Geometry: final body of the model. Coordinates: model frame, mm. Face numbers are marked on the shaded views. A direction names the side the tool comes from. Give positions to 0.01 mm unless a question says otherwise; leave off trailing zeros. Write each loop counter-clockwise with the first axis right and the second up, starting at its lowest first coordinate (ties: lowest second). Pieces come first, ordered by that corner, then holes.
Q1. Section C-C (z = -1.5). Return the cut outline in (x, y).
Q2. Pin query (flat end, axial travel): pin 1 Ø12 at (x, y) = (74, -29.5) entering from +Z; pin 2 Ø6 at (y, z) = (-23, -5) entering from +X; pin 3 Ø0.9 at (x, y) = (95.5, -13.5) entering from -Z. Return the tip coordinate at first contact, or that it passes through.
Q3. Section D-D (y = -25). Return the cut outline in (x, z) (3 decimals), plus the area to 3 significant figures.
Q4. Section B-B (x = 55.5). Return the cut outline in (y, z).
Q5. Reachability of the marked faces 1 and 2 from +Z, -Z, +X, -X, +Y, -Y: full face, straight path, thin tool, end or side. Return the list, or none.
Q6. Line query: line 1 (Z direction, x = 44.5, y = -6.5); line 2 (Y direction, x = 22, z = -9.5); line 3 (Z direction, x = 97, y = -20). Output: solid intervals per line, ascending.
Q7. Section A-A (y = -53.5). Return the cut outline in (x, z), plus the area to 3 significant figures.
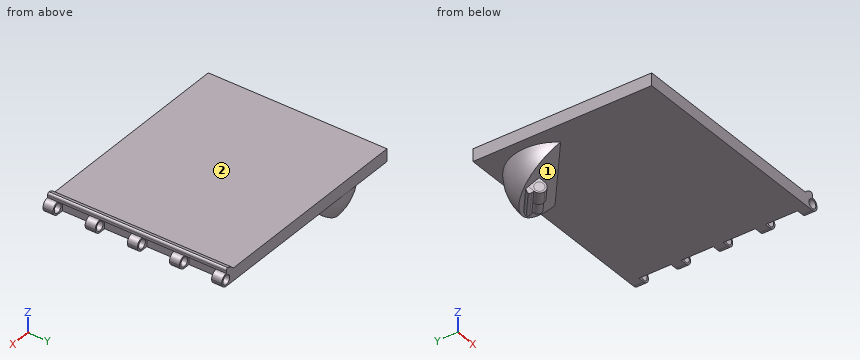
from build123d import *

# Parameters (mm, degrees)
F0_W      = 100
F0_H      = 5.6
F1_DEPTH  = 80
F3_R      = 2.05
F4_DEPTH  = 80
F2_W      = 5.7
F2_H      = 14.37
F2_W_2    = 5.6900524584
F2_W_3    = 5.6801049167
F2_W_4    = 5.6701573751
F5_DEPTH  = 5.6
F6_DEPTH  = 80
F8_ANGLE  = 45
F10_DEPTH = 5.6
F12_DEPTH = 7.185
F11_R     = 2.05
F13_DEPTH = 14.37


with BuildPart() as f1:
    # F0 (on Front) → F1 (new body)
    with BuildSketch(Plane.XZ):
        with Locations((50, 2.8)):
            Rectangle(F0_W, F0_H)
    extrude(amount=F1_DEPTH)

    # F3 (on face) → F4 (cut)
    with BuildSketch(Plane(origin=(0, 0, 0), x_dir=(-1, 0, 0), z_dir=(0, 1, 0))):
        with BuildLine():
            ThreePointArc((-100, 2.8), (-99.1798989873, 4.7798989873), (-97.2, 5.6))
            Line((-97.2, 5.6), (-100, 5.6))
            Line((-100, 5.6), (-100, 2.8))
        make_face()
        with BuildLine():
            ThreePointArc((-97.2, 0), (-99.1798989873, 0.8201010127), (-100, 2.8))
            Line((-100, 2.8), (-100, 0))
            Line((-100, 0), (-97.2, 0))
        make_face()
        with Locations((-97.2, 2.8)):
            Circle(F3_R)
    extrude(amount=-F4_DEPTH, mode=Mode.SUBTRACT)

    # F2 (on face) → F5 (cut)
    with BuildSketch(Plane.XY.offset(5.6)):
        with Locations((97.15, -11.689)):
            Rectangle(F2_W, F2_H)
        with Locations((97.1549737708, -30.5629973786)):
            Rectangle(F2_W_2, F2_H)
        with Locations((97.1599475416, -49.4369947571)):
            Rectangle(F2_W_3, F2_H)
        with Locations((97.1649213125, -68.3109921357)):
            Rectangle(F2_W_4, F2_H)
    extrude(amount=-F5_DEPTH, mode=Mode.SUBTRACT)

    # F3 (on face) → F6 (join)
    with BuildSketch(Plane(origin=(0, 0, 0), x_dir=(-1, 0, 0), z_dir=(0, 1, 0))):
        with BuildLine():
            ThreePointArc((-96.4487730361, 7.7432436768), (-96.9926506427, 7.3427867688), (-97.2, 6.7))
            ThreePointArc((-97.2, 6.7), (-96.8778174593, 5.9221825407), (-96.1, 5.6))
            Line((-96.1, 5.6), (-94.4, 5.6))
            Line((-94.4, 5.6), (-93.0575369646, 5.6))
            ThreePointArc((-93.0575369646, 5.6), (-94.5287785908, 7.0266507051), (-96.4487730361, 7.7432436768))
        make_face()
        with BuildLine():
            ThreePointArc((-96.1, 5.6), (-96.8778174593, 5.9221825407), (-97.2, 6.7))
            Line((-97.2, 6.7), (-97.2, 5.6))
            Line((-97.2, 5.6), (-96.1, 5.6))
        make_face()
    extrude(amount=-F6_DEPTH)

    # F7 (on face) → F8 (revolve)
    with BuildSketch(Plane(origin=(0, 0, 0), x_dir=(1, 0, 0), z_dir=(0, 0, -1))):
        with BuildLine():
            Line((39.6402182962, 7.3743059291), (8.9597817038, 32.6256940709))
            ThreePointArc((8.9597817038, 32.6256940709), (11.6743059291, 4.6597817038), (39.6402182962, 7.3743059291))
        make_face()
    revolve(axis=Axis((24.3, -20, 0), (-0.7721136423, -0.6354844793, 0)), revolution_arc=F8_ANGLE)

    # F9 (on face) → F10 (join)
    with BuildSketch(Plane(origin=(9.8133247181, -11.9231895325, -15.442272846), x_dir=(0.8933530871, 0.274620552, 0.3556737467), z_dir=(0.4493553846, -0.5459667923, -0.7071067812))):
        Polygon((8.4025323119, 2.4046372142), (11.2193246755, 7.2446455593), (5.0094211114, 10.8586907615), (2.1926287478, 6.0186824164), align=None)
    extrude(amount=F10_DEPTH)

    # F11 (on face) → F12 (cut)
    with BuildSketch(Plane(origin=(-0.874285956, -0.7195769186, 0), x_dir=(0.6354844793, -0.7721136423, 0), z_dir=(-0.7721136423, -0.6354844793, 0))):
        with BuildLine():
            ThreePointArc((25.8401079833, -12.9640336579), (23.8602089959, -13.7841346706), (21.8803100086, -12.9640336579))
            Line((21.8803100086, -12.9640336579), (23.8602089959, -14.9439326453))
            Line((23.8602089959, -14.9439326453), (25.8401079833, -12.9640336579))
        make_face()
        with BuildLine():
            Line((27.8200069706, -10.9841346706), (25.8401079833, -9.0042356833))
            ThreePointArc((25.8401079833, -9.0042356833), (26.447071687, -9.91262106), (26.6602089959, -10.9841346706))
            ThreePointArc((26.6602089959, -10.9841346706), (26.447071687, -12.0556482812), (25.8401079833, -12.9640336579))
            Line((25.8401079833, -12.9640336579), (27.8200069706, -10.9841346706))
        make_face()
    extrude(amount=-F12_DEPTH, mode=Mode.SUBTRACT)

    # F11 (on face) → F13 (join)
    with BuildSketch(Plane(origin=(-0.874285956, -0.7195769186, 0), x_dir=(0.6354844793, -0.7721136423, 0), z_dir=(-0.7721136423, -0.6354844793, 0))):
        with BuildLine():
            ThreePointArc((21.1024925493, -12.1862161986), (19.9483442634, -11.9304113338), (19.228840788, -12.8683927535))
            ThreePointArc((19.228840788, -12.8683927535), (19.4976789162, -13.4271515153), (19.8336101906, -13.9483381152))
            ThreePointArc((19.8336101906, -13.9483381152), (20.5013555296, -14.0497518637), (21.1024925493, -13.7418511172))
            ThreePointArc((21.1024925493, -13.7418511172), (21.42467509, -12.9640336579), (21.1024925493, -12.1862161986))
        make_face()
        with BuildLine():
            Line((19.9004110213, -10.9841346706), (18.8602089959, -10.9841346706))
            ThreePointArc((18.8602089959, -10.9841346706), (18.9532322771, -11.9441239832), (19.228840788, -12.8683927535))
            ThreePointArc((19.228840788, -12.8683927535), (19.9483442634, -11.9304113338), (21.1024925493, -12.1862161986))
            Line((21.1024925493, -12.1862161986), (19.9004110213, -10.9841346706))
        make_face()
        with BuildLine():
            Line((21.8803100086, -12.9640336579), (21.1024925493, -12.1862161986))
            ThreePointArc((21.1024925493, -12.1862161986), (21.42467509, -12.9640336579), (21.1024925493, -13.7418511172))
            Line((21.1024925493, -13.7418511172), (21.8803100086, -12.9640336579))
        make_face()
        with Locations((23.8602089959, -10.9841346706)):
            Circle(F11_R)
    extrude(amount=-F13_DEPTH)


solid = f1.part
Computed:
1. outline: (8.09, -31.4) - (38.6, -6.29) arc R19.81 ccw to start
2. pin 1: stops at z = 5.6
2. pin 2: stops at x = 18.75
2. pin 3: stops at z = 5.6
3. outline: (0, 0) - (5.072, 0) arc R19.228 ccw to (6.558, -7.414) - (18.225, 0) - (94.31, 0) - (94.31, 5.6) - (97.2, 5.6) - (97.2, 6.7) arc R1.1 ccw to (96.449, 7.743) arc R5 ccw to (93.058, 5.6) - (0, 5.6) - close
3. area: 585 mm2
4. outline: (-80, 0) - (0, 0) - (0, 5.6) - (-80, 5.6) - close
5. face 1: none
5. face 2: +Z, -X, +Y, -Y
6. line 1: z = 0 to 5.6
6. line 2: y = -14.63 to -10.96, -9.59 to -2.7
6. line 3: z = 0 to 0.76, 4.84 to 7.33
7. outline: (0, 0) - (94.32, 0) - (94.32, 5.6) - (97.2, 5.6) - (97.2, 6.7) arc R1.1 ccw to (96.45, 7.74) arc R5 ccw to (93.06, 5.6) - (0, 5.6) - close
7. area: 534 mm2
